For this review, take the finished solid that the model builds, in its own axes (mm). Round coordinates to 2 decimals unless told otherwise and drop trailing zeros. Loops run counter-clockwise (first coordinate to the right, second up) from the corner with the lowest first, then second, coordinate; pieces in that order, holes last.
1. Consider section A-A on x = -10. State the section outline as (y, z) points, then the cut area to 4 significant figures.
2. To check wall thickness, follow line 1 along Z through (x, y) = (-105.5, 1.5); line 2 along X through (y, z) = (2.2, -19); line 3 along X through (y, z) = (0.5, -80). State the ranges of each line that lie inside material, in increasing order.
3. Consider section B-B on y = 2. State the section outline as (x, z) points.
4. Consider section C-C on x = -105. State the section outline as (y, z) points, then the cut area to 3 significant figures.
5. Clearance check with flat-ended pins moving along their axes: pin 1 Ø0.8 at (y, z) = (1, -57) entering from -X; pin 2 Ø0.8 at (y, z) = (1, -39) entering from +X; pin 3 Ø0.8 at (y, z) = (1.5, -9.5) entering from +X. State where each tip first meets the part, or that it passes through.
6. Consider section D-D on z = -33.5. State the section outline as (x, y) points.
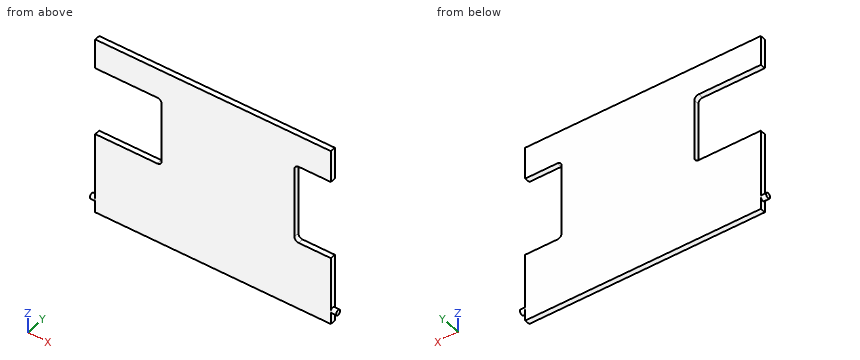
from build123d import *

# Parameters (mm, degrees)
CROQUIS1_W              = 110
CROQUIS1_H              = 84
SALIENTE_EXTRUIR1_DEPTH = 2.5
CROQUIS2_R              = 1.25
SALIENTE_EXTRUIR2_DEPTH = 2.5
CROQUIS3_R              = 1.25
SALIENTE_EXTRUIR3_DEPTH = 2.5
CORTAR_EXTRUIR1_DEPTH   = 10


with BuildPart() as part:
    # Croquis1 → Saliente-Extruir1 (new body)
    with BuildSketch(Plane(origin=(0, 0, 0), x_dir=(1, 0, 0), z_dir=(0, 1, 0))):
        with Locations((-55, 42)):
            Rectangle(CROQUIS1_W, CROQUIS1_H)
    extrude(amount=SALIENTE_EXTRUIR1_DEPTH)

    # Croquis2 → Saliente-Extruir2 (add)
    with BuildSketch(Plane(origin=(0, 0, 0), x_dir=(0, 0, -1), z_dir=(1, 0, 0))):
        with Locations((78, 1.25)):
            Circle(CROQUIS2_R)
    extrude(amount=SALIENTE_EXTRUIR2_DEPTH)

    # Croquis3 → Saliente-Extruir3 (add)
    with BuildSketch(Plane.ZY.offset(110)):
        with Locations((-78, 1.25)):
            Circle(CROQUIS3_R)
    extrude(amount=SALIENTE_EXTRUIR3_DEPTH)

    # Croquis4 → Cortar-Extruir1 (cut)
    with BuildSketch(Plane(origin=(0, 2.5, 0), x_dir=(1, 0, 0), z_dir=(0, 1, 0))):
        with BuildLine():
            Line((-81, 46), (-110, 46))
            Line((-110, 46), (-110, 14))
            Line((-110, 14), (-81, 14))
            ThreePointArc((-81, 14), (-79.585786438, 14.585786438), (-79, 16))
            Line((-79, 16), (-79, 44))
            ThreePointArc((-79, 44), (-79.585786438, 45.414213562), (-81, 46))
        make_face()
        with BuildLine():
            Line((-17, 17), (-17, 50))
            ThreePointArc((-17, 50), (-16.414213562, 51.414213562), (-15, 52))
            Line((-15, 52), (0, 52))
            Line((0, 52), (0, 15))
            Line((0, 15), (-15, 15))
            ThreePointArc((-15, 15), (-16.414213562, 15.585786438), (-17, 17))
        make_face()
    extrude(amount=-CORTAR_EXTRUIR1_DEPTH, mode=Mode.SUBTRACT)


solid = part.part
Resolved:
1. outline: (0, -84) - (2.5, -84) - (2.5, -52) - (0, -52) - close; (0, -15) - (2.5, -15) - (2.5, 0) - (0, 0) - close
1. area: 117.5 mm2
2. line 1: z = -84 to -46, -14 to 0
2. line 2: x = -79 to -17
2. line 3: x = -110 to 0
3. outline: (-112.5, -79) - (-110, -79) - (-110, -84) - (0, -84) - (0, -79) - (2.5, -79) - (2.5, -77) - (0, -77) - (0, -52) - (-15, -52) arc R2 cw to (-17, -50) - (-17, -17) arc R2 cw to (-15, -15) - (0, -15) - (0, 0) - (-110, 0) - (-110, -14) - (-81, -14) arc R2 cw to (-79, -16) - (-79, -44) arc R2 cw to (-81, -46) - (-110, -46) - (-110, -77) - (-112.5, -77) - close
4. outline: (0, -84) - (2.5, -84) - (2.5, -46) - (0, -46) - close; (0, -14) - (2.5, -14) - (2.5, 0) - (0, 0) - close
4. area: 130 mm2
5. pin 1: stops at x = -110
5. pin 2: stops at x = -17
5. pin 3: stops at x = 0
6. outline: (-79, 0) - (-17, 0) - (-17, 2.5) - (-79, 2.5) - close
